from build123d import *

# Parameters (mm, degrees)
ESTRUSIONE_ESTRUSIONE2_DEPTH      = 1
ESTRUSIONE_ESTRUSIONE2_2_DEPTH    = 1
ESTRUSIONE_ESTRUSIONE3_DEPTH      = 15
SCHIZZO4_W                        = 100
SCHIZZO4_H                        = 70
SCHIZZO4_R                        = 3.4
ESTRUSIONE_ESTRUSIONE4_DEPTH      = 20
SCHIZZO5_R                        = 2.5
TAGLIO_ESTRUSIONE2_DEPTH          = 36
SCHIZZO6_R                        = 5
TAGLIO_ESTRUSIONE3_DEPTH          = 10
SCHIZZO7_R                        = 6
TAGLIO_ESTRUSIONE4_DEPTH          = 8
RACCORDO1_R                       = 1
RACCORDO2_R                       = 1
ESTRUSIONE_ESTRUSIONE5_DEPTH      = 20
RACCORDO3_R                       = 10
ESTRUSIONE_ESTRUSIONE6_DEPTH      = 30
SCHIZZO11_W                       = 20
SCHIZZO11_H                       = 5
ESTRUSIONE_ESTRUSIONE7_DEPTH      = 17.5
ESTRUSIONE_ESTRUSIONE7_DEPTH_BACK = 47.5
TAGLIO_ESTRUSIONE5_REACH          = 192
SCHIZZO13_R                       = 2.5


with BuildPart() as part:
    # Schizzo1 → Estrusione-Estrusione2 (new body)
    with BuildSketch(Plane.XY):
        with BuildLine():
            ThreePointArc((-1482, 0), (-1485, 3), (-1488, 0))
            ThreePointArc((-1488, 0), (-1485, -3), (-1482, 0))
        make_face()
    extrude(amount=-ESTRUSIONE_ESTRUSIONE2_DEPTH)



with BuildPart() as body_2:
    # Schizzo1 → Estrusione-Estrusione2 2 (new body)
    with BuildSketch(Plane.XY):
        with BuildLine():
            ThreePointArc((-1475.75, 0), (-1460, -15.75), (-1444.25, 0))
            ThreePointArc((-1444.25, 0), (-1460, 15.75), (-1475.75, 0))
        make_face()
    extrude(amount=-ESTRUSIONE_ESTRUSIONE2_2_DEPTH)


with BuildPart() as part_1:
    add(part.part)

    add(body_2.part)  # Estrusione-Estrusione3 merges body 2
    # Schizzo2 → Estrusione-Estrusione3 (add)
    with BuildSketch(Plane.XY):
        with BuildLine():
            ThreePointArc((-1491.5, 0), (-1460, -31.5), (-1428.5, 0))
            ThreePointArc((-1428.5, 0), (-1460, 31.5), (-1491.5, 0))
        make_face()
        with BuildLine():
            ThreePointArc((-1479.150635095, -12.5), (-1481.650635095, -10), (-1484.150635095, -12.5))
            ThreePointArc((-1484.150635095, -12.5), (-1481.650635095, -15), (-1479.150635095, -12.5))
        make_face(mode=Mode.SUBTRACT)
        with BuildLine():
            ThreePointArc((-1457.5, -25), (-1460, -22.5), (-1462.5, -25))
            ThreePointArc((-1462.5, -25), (-1460, -27.5), (-1457.5, -25))
        make_face(mode=Mode.SUBTRACT)
        with BuildLine():
            ThreePointArc((-1435.849364905, -12.5), (-1438.349364905, -10), (-1440.849364905, -12.5))
            ThreePointArc((-1440.849364905, -12.5), (-1438.349364905, -15), (-1435.849364905, -12.5))
        make_face(mode=Mode.SUBTRACT)
        with BuildLine():
            ThreePointArc((-1435.849364905, 12.5), (-1438.349364905, 15), (-1440.849364905, 12.5))
            ThreePointArc((-1440.849364905, 12.5), (-1438.349364905, 10), (-1435.849364905, 12.5))
        make_face(mode=Mode.SUBTRACT)
        with BuildLine():
            ThreePointArc((-1462.5, 25), (-1460, 22.5), (-1457.5, 25))
            ThreePointArc((-1457.5, 25), (-1460, 27.5), (-1462.5, 25))
        make_face(mode=Mode.SUBTRACT)
        with BuildLine():
            ThreePointArc((-1479.150635095, 12.5), (-1481.650635095, 15), (-1484.150635095, 12.5))
            ThreePointArc((-1484.150635095, 12.5), (-1481.650635095, 10), (-1479.150635095, 12.5))
        make_face(mode=Mode.SUBTRACT)
    extrude(amount=ESTRUSIONE_ESTRUSIONE3_DEPTH)

    # Schizzo4 → Estrusione-Estrusione4 (add)
    with BuildSketch(Plane.XY.offset(15)):
        with Locations((-1460, 0)):
            Rectangle(SCHIZZO4_W, SCHIZZO4_H)
        with Locations((-1501, 22.5)):
            Circle(SCHIZZO4_R, mode=Mode.SUBTRACT)
        with Locations((-1419, -22.5)):
            Circle(SCHIZZO4_R, mode=Mode.SUBTRACT)
        with Locations((-1419, 22.5)):
            Circle(SCHIZZO4_R, mode=Mode.SUBTRACT)
        with Locations((-1501, -22.5)):
            Circle(SCHIZZO4_R, mode=Mode.SUBTRACT)
    extrude(amount=ESTRUSIONE_ESTRUSIONE4_DEPTH)

    # Schizzo5 → Taglio-Estrusione2 (cut)
    with BuildSketch(Plane(origin=(0, 0, -1), x_dir=(-1, 0, 0), z_dir=(0, 0, -1))):
        with Locations((1438.349364905, 12.5)):
            Circle(SCHIZZO5_R)
        with Locations((1438.349364905, -12.5)):
            Circle(SCHIZZO5_R)
        with Locations((1460, -25)):
            Circle(SCHIZZO5_R)
        with Locations((1481.650635095, -12.5)):
            Circle(SCHIZZO5_R)
        with Locations((1481.650635095, 12.5)):
            Circle(SCHIZZO5_R)
        with Locations((1460, 25)):
            Circle(SCHIZZO5_R)
    extrude(amount=-TAGLIO_ESTRUSIONE2_DEPTH, mode=Mode.SUBTRACT)

    # Schizzo6 → Taglio-Estrusione3 (cut)
    with BuildSketch(Plane.XY.offset(35)):
        with Locations((-1460, 25)):
            Circle(SCHIZZO6_R)
        with Locations((-1438.349364905, 12.5)):
            Circle(SCHIZZO6_R)
        with Locations((-1438.349364905, -12.5)):
            Circle(SCHIZZO6_R)
        with Locations((-1460, -25)):
            Circle(SCHIZZO6_R)
        with Locations((-1481.650635095, -12.5)):
            Circle(SCHIZZO6_R)
        with Locations((-1481.650635095, 12.5)):
            Circle(SCHIZZO6_R)
    extrude(amount=-TAGLIO_ESTRUSIONE3_DEPTH, mode=Mode.SUBTRACT)

    # Schizzo7 → Taglio-Estrusione4 (cut)
    with BuildSketch(Plane(origin=(0, 0, 15), x_dir=(-1, 0, 0), z_dir=(0, 0, -1))):
        with Locations((1419, 22.5)):
            Circle(SCHIZZO7_R)
        with Locations((1501, -22.5)):
            Circle(SCHIZZO7_R)
        with Locations((1501, 22.5)):
            Circle(SCHIZZO7_R)
        with Locations((1419, -22.5)):
            Circle(SCHIZZO7_R)
    extrude(amount=-TAGLIO_ESTRUSIONE4_DEPTH, mode=Mode.SUBTRACT)

    # Raccordo1
    raccordo1_edges = [part_1.edges().sort_by_distance(p)[0] for p in [
        (-1510, 35, 25),
        (-1510, -35, 25),
        (-1410, -35, 25),
        (-1410, 35, 25),
    ]]
    fillet(raccordo1_edges, radius=RACCORDO1_R)

    # Raccordo2
    raccordo2_edges = [part_1.edges().sort_by_distance(p)[0] for p in [
        (-1491.5, 0, 15),
    ]]
    fillet(raccordo2_edges, radius=RACCORDO2_R)

    # Schizzo8 → Estrusione-Estrusione5 (add)
    with BuildSketch(Plane.XY.offset(35)):
        Polygon((-1460, -35), (-1475, -35), (-1475, -155), (-1465.76, -155), (-1445, -155), (-1445, -35), align=None)
    extrude(amount=-ESTRUSIONE_ESTRUSIONE5_DEPTH)

    # Raccordo3
    raccordo3_edges = [part_1.edges().sort_by_distance(p)[0] for p in [
        (-1445, -35, 25),
        (-1475, -35, 25),
    ]]
    fillet(raccordo3_edges, radius=RACCORDO3_R)

    # Schizzo10 → Estrusione-Estrusione6 (add)
    with BuildSketch(Plane.ZY.offset(1475)):
        Polygon((20.7, -155), (20.7, -156.76), (16.7, -156.76), (16.7, -160.36), (20.483021279, -164.143021279), (29.516978721, -164.143021279), (33.3, -160.36), (33.3, -156.76), (29.3, -156.76), (29.3, -155), align=None)
    extrude(amount=-ESTRUSIONE_ESTRUSIONE6_DEPTH)

    # Schizzo11 → Estrusione-Estrusione7 (add, two sides)
    with BuildSketch(Plane(origin=(-1445, 0, 0), x_dir=(0, 0, -1), z_dir=(1, 0, 0))) as estrusione_estrusione7_sk:
        with Locations((-25, -152.5)):
            Rectangle(SCHIZZO11_W, SCHIZZO11_H)
    extrude(amount=ESTRUSIONE_ESTRUSIONE7_DEPTH)
    extrude(estrusione_estrusione7_sk.sketch, amount=-ESTRUSIONE_ESTRUSIONE7_DEPTH_BACK)

    # Schizzo13 → Taglio-Estrusione5 (cut, up to next)
    with BuildSketch(Plane.XZ.offset(155), mode=Mode.PRIVATE) as taglio_estrusione5_sk1:
        with Locations((-1437.15, 25)):
            Circle(SCHIZZO13_R)
    taglio_estrusione5_tool1 = extrude(taglio_estrusione5_sk1.sketch, amount=-TAGLIO_ESTRUSIONE5_REACH, mode=Mode.PRIVATE) & part_1.part
    add(taglio_estrusione5_tool1.solids().sort_by_distance((-1437.15, -155, 25))[0], mode=Mode.SUBTRACT)
    # Schizzo13 → Taglio-Estrusione5 (cut, up to next)
    with BuildSketch(Plane.XZ.offset(155), mode=Mode.PRIVATE) as taglio_estrusione5_sk2:
        with Locations((-1482.85, 25)):
            Circle(SCHIZZO13_R)
    taglio_estrusione5_tool2 = extrude(taglio_estrusione5_sk2.sketch, amount=-TAGLIO_ESTRUSIONE5_REACH, mode=Mode.PRIVATE) & part_1.part
    add(taglio_estrusione5_tool2.solids().sort_by_distance((-1482.85, -155, 25))[0], mode=Mode.SUBTRACT)


solid = part_1.part
Here's how the part is built. I have some questions about the finished solid (model axes, mm). A direction names the side the tool comes from. Give positions to 0.01 mm unless a question says otherwise; leave off trailing zeros. Order: outer loops, then holes, each group sorted by start corner. A loop starts at its lowest first (then second) coordinate and runs counter-clockwise, first axis right, second up. Notation, with made-up numbers: (30.25, 80.25) -> (82.25, 80.25) arc R26 ccw to (82.25, 95.25) -> close; hole circle Ø5 at (38.5, 19). An arc over 180 degrees is marked (long way). One line per item, written item: value. Start each with the question number.
1. Imagine slicing it at D-D, the plane y = -12.5. Count the separate pieces of the cut face and the enclosed holes in it, plus the area to 3 significant figures.
2. Imagine slicing it at A-A, the plane x = -1419. List the corners of the cut face in (y, z) for me, plus the area to 3 significant figures.
3. Imagine slicing it at B-B, the plane z = 7. List the corners of the cut face in (x, y) for me.
4. For faces 4 (the face through (-1434.765, -152.535, 25.751)), 5 (the face through (-1467.4, 14.4, 0)), 6 (the face through (-1475, -160, 25)), 7 (the face through (-1445, -160, 25)), 8 (the face through (-1478.01, -37.85, 24.86)), which set-ups out of +Z, -Z, +X, -X, +Y, -Y let a thin tool reach every point of the face, with its end or its side?
5. I need wall thicknesses on probe 1 along X at (y, z) = (-22, 17); probe 2 along X at (y, z) = (22.5, 30.5); probe 3 along Y at (x, z) = (-1501, 30). Which ranges of each line are inside material? Lowest first, please. Write a range as from..to.
6. Imagine slicing it at C-C, the plane y = -128. List the corners of the cut face in (x, z) for me.
7. Will these pins go through, and if not, where does the flat tip stop? pin 1 Ø6 at (y, z) = (-117, 13.5) entering from +X; pin 2 Ø5 at (y, z) = (-39, 18) entering from -X; pin 3 Ø2.5 at (y, z) = (-159.5, 21) entering from -X; pin 4 Ø8 at (x, y) = (-1438, -109) entering from -Z.
8. We'd pull the mould along Z, two halves only. Please class faces 1 (the face through (-1460, -156.76, 19)), 2 (the face through (-1480.465, -152.535, 25.751)), 3 (the face through (-1504, -25, 23)): released by +Z, released by -Z, zero draft, split by the parting line, or undercut.
Values follow:
1. separate pieces: 3
1. enclosed holes: 0
1. area: 2,440 mm2
2. outline: (-35, 15) -> (-28.5, 15) -> (-28.5, 23) -> (-25.9, 23) -> (-25.9, 35) -> (-35, 35) -> close; (-19.1, 23) -> (-16.5, 23) -> (-16.5, 15) -> (16.5, 15) -> (16.5, 23) -> (19.1, 23) -> (19.1, 35) -> (-19.1, 35) -> close; (25.9, 23) -> (28.5, 23) -> (28.5, 15) -> (35, 15) -> (35, 35) -> (25.9, 35) -> close
2. area: 1,040 mm2
3. outline: circle Ø63 at (-1460, 0); hole circle Ø5 at (-1481.65, -12.5); hole circle Ø5 at (-1481.65, 12.5); hole circle Ø5 at (-1460, -25); hole circle Ø5 at (-1460, 25); hole circle Ø5 at (-1438.35, -12.5); hole circle Ø5 at (-1438.35, 12.5)
4. face 4: -Y
4. face 5: -Z
4. face 6: +Z, -Z, -X, -Y
4. face 7: +Z, -Z, +X, -Y
4. face 8: +Z, -Z, -X
5. probe 1: x = -1510..-1506.98, -1495.02..-1424.98, -1413.02..-1410
5. probe 2: x = -1510..-1504.4, -1497.6..-1464.33, -1455.67..-1422.4, -1415.6..-1410
5. probe 3: y = -35..-25.9, -19.1..19.1, 25.9..35
6. outline: (-1475, 15) -> (-1445, 15) -> (-1445, 35) -> (-1475, 35) -> close
7. pin 1: stops at x = -1445
7. pin 2: stops at x = -1479.73
7. pin 3: stops at x = -1475
7. pin 4: passes through
8. face 1: zero draft
8. face 2: undercut
8. face 3: released by -Z
